Solid Edge part; units mm, degrees
sketch "Sketch1" plane through (0, 0, 0) normal (0, 0, 1) x (1, 0, 0)
  circle A0 centre (0, -19.925) radius 3.1
  circle A1 centre (0, 19.925) radius 3.1
  arc A2 (9, 29) -> (19, 19) centre (9, 19) cw
  line L0 (19, -29) -> (19, 19)
  line L1 (19, -41) -> (19, -29)
  line L2 (-19, -41) -> (19, -41)
  line L3 (-5.5, -41) -> (5.5, -41) construction
  line L4 (-19, -29) -> (-19, -41)
  line L5 (-19, 19) -> (-19, -29)
  arc A3 (-9, 29) -> (-19, 19) centre (-9, 19) ccw
  line L6 (9, 29) -> (-9, 29)
extrude "Protrusion1" add sketch "Sketch1" against normal blind 5
sketch "Sketch2" plane through (0, -41, -2.5) normal (0, -1, 0) x (1, 0, 0)
  line L0 (-19, -2.5) -> (19, -2.5)
  line L1 (19, -2.5) -> (19, 17.5)
  line L2 (19, 17.5) -> (19, 46)
  arc A0 (9.5, 55.5) -> (19, 46) centre (9.5, 46) cw
  line L3 (9.5, 55.5) -> (-9.5, 55.5)
  arc A1 (-9.5, 55.5) -> (-19, 46) centre (-9.5, 46) ccw
  line L4 (-19, 46) -> (-19, 17.5)
  line L5 (-19, 17.5) -> (-19, -2.5)
  circle A2 centre (-9.5, 27) radius 6.1
  circle A3 centre (9.5, 27) radius 6.1
  circle A4 centre (9.5, 46) radius 6.1
  circle A5 centre (-9.5, 46) radius 6.1
extrude "Extrusionsausprägung_2" add sketch "Sketch2" along normal blind 5
chamfer "Fase_1" distance 10 angle 45 1 edges at (0, -41, 0)
Can you work these out from the model? Positions are in its coordinate system, mm. A direction names the side the tool comes from. Round coordinates to 2 decimals unless told otherwise and drop trailing zeros. Order: outer loops, then holes, each group sorted by start corner. A loop starts at its lowest first (then second) coordinate and runs counter-clockwise, first axis right, second up.
(1) On a 3-axis mill with a long thin cutter (end or side, diameter ignored), from which of +Z, -Z, +X, -X, +Y, -Y can I reach the whole of each face in a straight line? I mean faces 1 (the face through (0, -41, 32)), 2 (the face through (16.15, 25.99, -2.46)). Say none if no direction works.
Results are:
face 1: +Z, +X, -X, +Y
face 2: +Z, -Z, +X, +Y
(2) We'd pull the mould along X, two halves only. Please class faces 3 (the face through (-15.99, 26.15, -2.46)), 4 (the face through (0, -36, 5)), 5 (the face through (-0.67, 16.9, -2.46)): +X half, -X half, draft (parallel to the pull), parting line (faces both ways), or undercut.
Results are:
face 3: -X half
face 4: draft
face 5: undercut
(3) If we section it at B-B (y = 21.5): Please give me the cut outline in (x, z), plus the area to 3 significant figures.
Results are:
outline: (-18.68, -5) - (-2.67, -5) - (-2.67, 0) - (-18.68, 0) - close; (2.67, -5) - (18.68, -5) - (18.68, 0) - (2.67, 0) - close
area: 160 mm2
(4) I'm going to push flat-ended pins straight in: pin 1 (12 mm diameter, centred on x = -6, y = -6.5, fed in from +Z); pin 2 (14 mm diameter, centred on x = -9.5, z = 24.5, fed in from +Y). Where does each tip first touch, or does it pass through?
Results are:
pin 1: stops at z = 0
pin 2: stops at y = -41
(5) If we section it at D-D (z = 1): Please give me the cut outline in (x, y), plus the area to 3 significant figures.
Results are:
outline: (-19, -46) - (19, -46) - (19, -32) - (-19, -32) - close
area: 532 mm2
(6) If I drill on L1, parallel to Z at x = -9.5, y = -44.15; L2, parallel to Y at x = 0, z = -2.5 (3 decimals); L3, parallel to X at y = -44, z = 43, over which ranges is the centre line in solid material (lowest first)?
Results are:
L1: z = -5 to 18.4, 30.6 to 37.4, 49.6 to 53
L2: y = -46 to -23.025, -16.825 to 16.825, 23.025 to 29
L3: x = -19 to -15.58, -3.42 to 3.42, 15.58 to 19
(7) If we section it at C-C (z = 24.5): Please give me the cut outline in (x, y), plus the area to 3 significant figures.
Results are:
outline: (-19, -46) - (-15.6, -46) - (-15.6, -41) - (-19, -41) - close; (-3.4, -46) - (3.4, -46) - (3.4, -41) - (-3.4, -41) - close; (15.6, -46) - (19, -46) - (19, -41) - (15.6, -41) - close
area: 68.0 mm2
(8) If we section it at A-A (x = 8): Please give me the cut outline in (y, z).
Results are:
outline: (-46, -5) - (29, -5) - (29, 0) - (-31, 0) - (-41, 10) - (-41, 18.59) - (-46, 18.59) - close; (-46, 30.41) - (-41, 30.41) - (-41, 37.59) - (-46, 37.59) - close; (-46, 49.41) - (-41, 49.41) - (-41, 53) - (-46, 53) - close
